```python
from build123d import *

# Parameters (mm, degrees)
SKETCH1_R           = 2.4892
BOSS_EXTRUDE1_DEPTH = 3.175


with BuildPart() as part:
    # Sketch1 → Boss-Extrude1 (new body)
    with BuildSketch(Plane.XY):
        with BuildLine():
            Line((33.978679656, -24.521320344), (37.221320344, -21.278679656))
            ThreePointArc((37.221320344, -21.278679656), (37.871638598, -20.30540961), (38.1, -19.157359313))
            Line((38.1, -19.157359313), (38.1, 19.157359313))
            ThreePointArc((38.1, 19.157359313), (37.871638598, 20.30540961), (37.221320344, 21.278679656))
            Line((37.221320344, 21.278679656), (33.978679656, 24.521320344))
            ThreePointArc((33.978679656, 24.521320344), (33.00540961, 25.171638598), (31.857359313, 25.4))
            Line((31.857359313, 25.4), (-31.857359313, 25.4))
            ThreePointArc((-31.857359313, 25.4), (-33.00540961, 25.171638598), (-33.978679656, 24.521320344))
            Line((-33.978679656, 24.521320344), (-37.221320344, 21.278679656))
            ThreePointArc((-37.221320344, 21.278679656), (-37.871638598, 20.30540961), (-38.1, 19.157359313))
            Line((-38.1, 19.157359313), (-38.1, -19.157359313))
            ThreePointArc((-38.1, -19.157359313), (-37.871638598, -20.30540961), (-37.221320344, -21.278679656))
            Line((-37.221320344, -21.278679656), (-33.978679656, -24.521320344))
            ThreePointArc((-33.978679656, -24.521320344), (-33.00540961, -25.171638598), (-31.857359313, -25.4))
            Line((-31.857359313, -25.4), (31.857359313, -25.4))
            ThreePointArc((31.857359313, -25.4), (33.00540961, -25.171638598), (33.978679656, -24.521320344))
        make_face()
        with Locations((13.470384182, 0)):
            Circle(SKETCH1_R, mode=Mode.SUBTRACT)
        with Locations((-25.4, 12.7)):
            Circle(SKETCH1_R, mode=Mode.SUBTRACT)
        with Locations((25.4, 12.7)):
            Circle(SKETCH1_R, mode=Mode.SUBTRACT)
        with Locations((25.4, -12.7)):
            Circle(SKETCH1_R, mode=Mode.SUBTRACT)
        with Locations((0, -12.7)):
            Circle(SKETCH1_R, mode=Mode.SUBTRACT)
        with Locations((-25.4, -12.7)):
            Circle(SKETCH1_R, mode=Mode.SUBTRACT)
        with Locations((0, 12.7)):
            Circle(SKETCH1_R, mode=Mode.SUBTRACT)
        Circle(SKETCH1_R, mode=Mode.SUBTRACT)
        with Locations((-13.470384182, 0)):
            Circle(SKETCH1_R, mode=Mode.SUBTRACT)
        with BuildLine():
            Line((11.2851302, -7.7648698), (14.4601302, -10.9398698))
            ThreePointArc((14.4601302, -10.9398698), (14.4601302, -14.4601302), (10.9398698, -14.4601302))
            Line((10.9398698, -14.4601302), (7.7648698, -11.2851302))
            ThreePointArc((7.7648698, -11.2851302), (7.7648698, -7.7648698), (11.2851302, -7.7648698))
        make_face(mode=Mode.SUBTRACT)
        with BuildLine():
            Line((-10.9398698, 14.4601302), (-7.7648698, 11.2851302))
            ThreePointArc((-7.7648698, 11.2851302), (-7.7648698, 7.7648698), (-11.2851302, 7.7648698))
            Line((-11.2851302, 7.7648698), (-14.4601302, 10.9398698))
            ThreePointArc((-14.4601302, 10.9398698), (-14.4601302, 14.4601302), (-10.9398698, 14.4601302))
        make_face(mode=Mode.SUBTRACT)
        with BuildLine():
            Line((-7.7648698, -11.2851302), (-10.9398698, -14.4601302))
            ThreePointArc((-10.9398698, -14.4601302), (-14.4601302, -14.4601302), (-14.4601302, -10.9398698))
            Line((-14.4601302, -10.9398698), (-11.2851302, -7.7648698))
            ThreePointArc((-11.2851302, -7.7648698), (-7.7648698, -7.7648698), (-7.7648698, -11.2851302))
        make_face(mode=Mode.SUBTRACT)
        with BuildLine():
            Line((14.4601302, 10.9398698), (11.2851302, 7.7648698))
            ThreePointArc((11.2851302, 7.7648698), (7.7648698, 7.7648698), (7.7648698, 11.2851302))
            Line((7.7648698, 11.2851302), (10.9398698, 14.4601302))
            ThreePointArc((10.9398698, 14.4601302), (14.4601302, 14.4601302), (14.4601302, 10.9398698))
        make_face(mode=Mode.SUBTRACT)
    extrude(amount=-BOSS_EXTRUDE1_DEPTH)


solid = part.part
```
Work out the finished part from the listing and answer in its coordinate system (mm). A direction names the side the tool comes from. Coordinates: 2 decimals unless noted, no trailing zeros. Write each loop counter-clockwise with the first axis right and the second up, starting at its lowest first coordinate (ties: lowest second). Pieces come first, ordered by that corner, then holes.
Q1. A cutting plane is placed at C-C, the plane y = -1.5. Give the vertices of the cut face in (x, z) (3 decimals), then the cut area to 3 significant figures.
Q2. Determine the mould class of faces 3 (the face through (-7.73, 7.8, -1.57)), 4 (the face through (35.6, -22.9, -1.6)), 5 (the face through (-37.865, 20.321, -1.565)) for opening direction X: released by +X, released by -X, zero draft, split by the parting line, or undercut.
Q3. Which of the six approach directions +Z, -Z, +X, -X, +Y, -Y give full straight-line access (tool end or side, diameter ignored) to faces 1 (the face through (-9.33, -12.85, -1.57)), 2 (the face through (-33.021, -25.165, -1.565))?
Q4. A cutting plane is placed at A-A, the plane x = -12.7. Give the vertices of the cut face in (y, z) (3 decimals).
Q5. A cutting plane is placed at D-D, the plane y = 13.5. Give the vertices of the cut face in (x, z) (3 decimals), then the cut area to 3 significant figures.
Q6. A cutting plane is placed at B-B, the plane x = 25.4. Give the vertices of the cut face in (y, z) (3 decimals).
Q7. Find the intervals of material crossed by line 1 (Y direction, x = -25.4, z = -2); line 2 (Y direction, x = 0, z = -1.05); line 3 (Y direction, x = 26, z = -1.1), in increasing order.
Findings below:
1. outline: (-38.1, -3.175) - (-15.457, -3.175) - (-15.457, 0) - (-38.1, 0) - close; (-11.484, -3.175) - (-1.986, -3.175) - (-1.986, 0) - (-11.484, 0) - close; (1.986, -3.175) - (11.484, -3.175) - (11.484, 0) - (1.986, 0) - close; (15.457, -3.175) - (38.1, -3.175) - (38.1, 0) - (15.457, 0) - close
1. area: 204 mm2
2. face 3: undercut
2. face 4: released by +X
2. face 5: released by -X
3. face 1: +Z, -Z
3. face 2: +Z, -Z, -X, -Y
4. outline: (-25.4, -3.175) - (-15.189, -3.175) - (-15.189, 0) - (-25.4, 0) - close; (-9.18, -3.175) - (-2.367, -3.175) - (-2.367, 0) - (-9.18, 0) - close; (2.367, -3.175) - (9.18, -3.175) - (9.18, 0) - (2.367, 0) - close; (15.189, -3.175) - (25.4, -3.175) - (25.4, 0) - (15.189, 0) - close
5. outline: (-38.1, -3.175) - (-27.757, -3.175) - (-27.757, 0) - (-38.1, 0) - close; (-23.043, -3.175) - (-15.057, -3.175) - (-15.057, 0) - (-23.043, 0) - close; (-9.98, -3.175) - (-2.357, -3.175) - (-2.357, 0) - (-9.98, 0) - close; (2.357, -3.175) - (9.98, -3.175) - (9.98, 0) - (2.357, 0) - close; (15.057, -3.175) - (23.043, -3.175) - (23.043, 0) - (15.057, 0) - close; (27.757, -3.175) - (38.1, -3.175) - (38.1, 0) - (27.757, 0) - close
5. area: 165 mm2
6. outline: (-25.4, -3.175) - (-15.189, -3.175) - (-15.189, 0) - (-25.4, 0) - close; (-10.211, -3.175) - (10.211, -3.175) - (10.211, 0) - (-10.211, 0) - close; (15.189, -3.175) - (25.4, -3.175) - (25.4, 0) - (15.189, 0) - close
7. line 1: y = -25.4 to -15.19, -10.21 to 10.21, 15.19 to 25.4
7. line 2: y = -25.4 to -15.19, -10.21 to -2.49, 2.49 to 10.21, 15.19 to 25.4
7. line 3: y = -25.4 to -15.12, -10.28 to 10.28, 15.12 to 25.4
